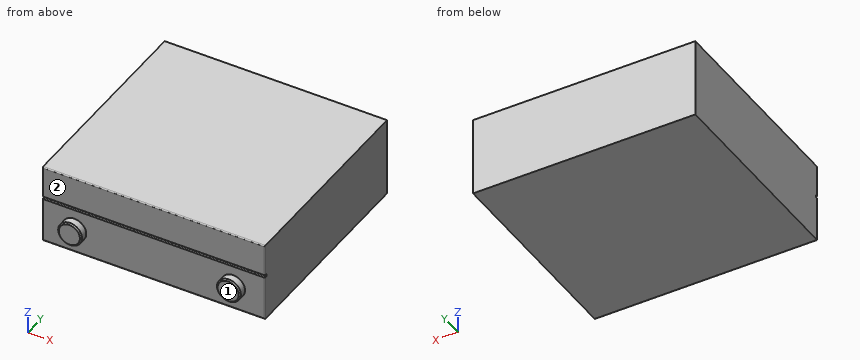
```python
from build123d import *

# Parameters (mm, degrees)
F0_W     = 420
F0_H     = 150
F1_DEPTH = 393
F2_R     = 2
F3_R     = 22.5
F4_DEPTH = 16
F5_SIZE  = 2.5
F6_W     = 5
F6_H     = 5
F7_DEPTH = 250


with BuildPart() as f1:
    # F0 (on Front) → F1 (new body)
    with BuildSketch(Plane.XZ):
        Rectangle(F0_W, F0_H)
    extrude(amount=-F1_DEPTH)

    # F2
    f2_edges = [f1.edges().sort_by_distance(p)[0] for p in [
        (210, 0, 0),
        (0, 0, 75),
        (-210, 0, 0),
        (0, 0, -75),
    ]]
    fillet(f2_edges, radius=F2_R)

    # F3 (on face) → F4 (join)
    with BuildSketch(Plane.XZ):
        with Locations((-150, -30)):
            Circle(F3_R)
        with Locations((150, -30)):
            Circle(F3_R)
    extrude(amount=F4_DEPTH)

    # F5
    f5_edges = [f1.edges().sort_by_distance(p)[0] for p in [
        (-172.5, -16, -30),
        (127.5, -16, -30),
    ]]
    chamfer(f5_edges, length=F5_SIZE)

    # F6 (on Right) → F7 (cut, symmetric)
    with BuildSketch(Plane.YZ):
        with Locations((2.5, 12.5)):
            Rectangle(F6_W, F6_H)
    extrude(amount=F7_DEPTH, both=True, mode=Mode.SUBTRACT)


solid = f1.part
```
Geometry: final body of the model. Coordinates: model frame, mm. Face numbers are marked on the shaded views. A direction names the side the tool comes from. Give positions to 0.01 mm unless a question says otherwise; leave off trailing zeros. Write each loop counter-clockwise with the first axis right and the second up, starting at its lowest first coordinate (ties: lowest second). Pieces come first, ordered by that corner, then holes.
1. Section query C-C, the plane x = -150. Return loops of the section in (y, z), then the cut area to 3 significant figures.
2. Reachability of the marked faces 1 and 2 from +Z, -Z, +X, -X, +Y, -Y: full face, straight path, thin tool, end or side. Return the list, or none.
3. Pin query (flat end, axial travel): P1, Ø4, axis at x = -14.5, z = -52, coming from the -Y side; P2, Ø1.5, axis at x = -76, z = 12, coming from the -Y side. Return the tip coordinate at first contact, or that it passes through.
4. Line query: probe 1 along Y at (x, z) = (-84.5, -40). Output: solid intervals per line, ascending.
5. Section query A-A, the plane x = -55. Return loops of the section in (y, z), then the cut area to 3 significant figures.
6. Section query D-D, the plane z = 61.5. Return loops of the section in (x, y).
7. Section query B-B, the plane z = -30. Return loops of the section in (x, y), then the cut area to 3 significant figures.
Computed:
1. outline: (-16, -50) - (-13.5, -52.5) - (0, -52.5) - (0, -73) arc R2 ccw to (2, -75) - (393, -75) - (393, 75) - (2, 75) arc R2 ccw to (0, 73) - (0, 15) - (5, 15) - (5, 10) - (0, 10) - (0, -7.5) - (-13.5, -7.5) - (-16, -10) - close
1. area: 59,600 mm2
2. face 1: +Z, -Z, +X, -X, -Y
2. face 2: +Z, +X, -X, -Y
3. P1: stops at y = 0
3. P2: stops at y = 5
4. probe 1: y = 0 to 393
5. outline: (0, -73) arc R2 ccw to (2, -75) - (393, -75) - (393, 75) - (2, 75) arc R2 ccw to (0, 73) - (0, 15) - (5, 15) - (5, 10) - (0, 10) - close
5. area: 58,900 mm2
6. outline: (-210, 2) arc R2 ccw to (-208, 0) - (208, 0) arc R2 ccw to (210, 2) - (210, 393) - (-210, 393) - close
7. outline: (-210, 2) arc R2 ccw to (-208, 0) - (-172.5, 0) - (-172.5, -13.5) - (-170, -16) - (-130, -16) - (-127.5, -13.5) - (-127.5, 0) - (127.5, 0) - (127.5, -13.5) - (130, -16) - (170, -16) - (172.5, -13.5) - (172.5, 0) - (208, 0) arc R2 ccw to (210, 2) - (210, 393) - (-210, 393) - close
7. area: 166,000 mm2
